Model file for the job. Use its own axes, mm. Face numbers are marked on the shaded views. A direction names the side the tool comes from. Give positions to 0.01 mm unless a question says otherwise; leave off trailing zeros. Loops run counter-clockwise (first coordinate to the right, second up) from the corner with the lowest first, then second, coordinate; pieces in that order, holes last. Notation, with made-up numbers: (23.5, 57.5) - (50.5, 57.5) arc R16 cw to (50.5, 67.5) - close; hole circle Ø2 at (50, -28). An arc over 180 degrees is marked (long way). Use a Markdown table: item, result.
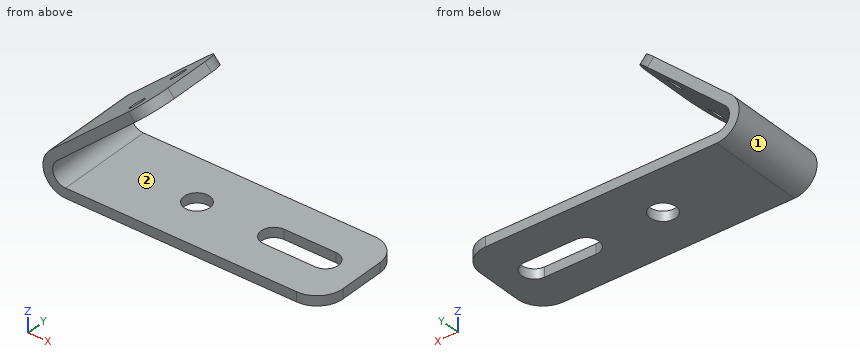
from build123d import *

# Parameters (mm, degrees)
F0_W          = 1270
F0_H          = 48.26
F1_DEPTH      = 483.87
F2_R          = 127
F3_R          = 127
F4_R          = 38.1
F5_DEPTH      = 119.38
F6_R          = 63.5
F7_DEPTH      = 76.2
F7_DEPTH_BACK = 76.2


with BuildPart() as f1:
    # F0 (on Front) → F1 (new body)
    with BuildSketch(Plane.XZ):
        with Locations((271.5897267231, -0.2383861614)):
            Rectangle(F0_W, F0_H)
        with BuildLine():
            Line((-363.4102732769, -24.3683861614), (-363.4102732769, 23.8916138386))
            ThreePointArc((-363.4102732769, 23.8916138386), (-423.8304438336, 67.7016554332), (-400.9706434856, 138.7463335075))
            Line((-400.9706434856, 138.7463335075), (-433.0378788647, 174.8118296935))
            ThreePointArc((-433.0378788647, 174.8118296935), (-468.9099911057, 50.5119834442), (-363.4102732769, -24.3683861614))
        make_face()
        Polygon((-433.0378788647, 174.8118296935), (-400.9706434856, 138.7463335075), (73.5753589619, 560.6836411268), (41.5081235828, 596.7491373128), align=None)
    extrude(amount=F1_DEPTH)

    # F2
    f2_edges = [f1.edges().sort_by_distance(p)[0] for p in [
        (57.541741, 0, 578.716389),
        (57.541741, -483.87, 578.716389),
    ]]
    fillet(f2_edges, radius=F2_R)

    # F3
    f3_edges = [f1.edges().sort_by_distance(p)[0] for p in [
        (906.589727, -483.87, -0.238386),
        (906.589727, 0, -0.238386),
    ]]
    fillet(f3_edges, radius=F3_R)

    # F4 (on face) → F5 (cut)
    with BuildSketch(Plane(origin=(-277.999987923, 0, 312.6620485248), x_dir=(0.7473165393, 0, 0.664468201), z_dir=(-0.664468201, 0, 0.7473165393))):
        with Locations((237.0405329721, -114.3)):
            Circle(F4_R)
        with Locations((237.0405329721, -369.57)):
            Circle(F4_R)
    extrude(amount=-F5_DEPTH, mode=Mode.SUBTRACT)

    # F6 (on face) → F7 (cut, two sides)
    with BuildSketch(Plane.XY.offset(23.8916138386)) as f7_sk:
        with Locations((93.7897267231, -241.935)):
            Circle(F6_R)
        with BuildLine():
            ThreePointArc((538.0487868786, -241.935), (519.4500674839, -197.0337193947), (474.5487868786, -178.435))
            ThreePointArc((474.5487868786, -178.435), (411.0487868786, -241.935), (474.5487868786, -305.435))
            ThreePointArc((474.5487868786, -305.435), (519.4500674839, -286.8362806053), (538.0487868786, -241.935))
        make_face()
        with BuildLine():
            ThreePointArc((729.6141386032, -305.435), (666.1141386032, -241.935), (729.6141386032, -178.435))
            Line((729.6141386032, -178.435), (474.5487868786, -178.435))
            ThreePointArc((474.5487868786, -178.435), (519.4500674839, -197.0337193947), (538.0487868786, -241.935))
            ThreePointArc((538.0487868786, -241.935), (519.4500674839, -286.8362806053), (474.5487868786, -305.435))
            Line((474.5487868786, -305.435), (729.6141386032, -305.435))
        make_face()
        with BuildLine():
            ThreePointArc((729.6141386032, -305.435), (774.5154192086, -286.8362806053), (793.1141386032, -241.935))
            ThreePointArc((793.1141386032, -241.935), (774.5154192086, -197.0337193947), (729.6141386032, -178.435))
            ThreePointArc((729.6141386032, -178.435), (666.1141386032, -241.935), (729.6141386032, -305.435))
        make_face()
    extrude(amount=-F7_DEPTH, mode=Mode.SUBTRACT)
    extrude(f7_sk.sketch, amount=F7_DEPTH_BACK, mode=Mode.SUBTRACT)


solid = f1.part
(1) Drill centre lines: probe 1 along Z at (x, y) = (591.5, -327); probe 2 along Z at (x, y) = (19.5, -57); probe 3 along Z at (x, y) = (-259, -419.5). Where is each one in solid material? Low to high. Write a range as [from, to].
Computed:
| item | result |
|---|---|
| probe 1 | [-24.37, 23.89] |
| probe 2 | [-24.37, 23.89], [512.6, 577.18] |
| probe 3 | [-24.37, 23.89], [264.98, 329.56] |
(2) Pin check, flat tips, straight feed: P1, Ø1, axis at y = -313, z = 426.5, coming from the +X side; P2, Ø1.5, axis at y = -166, z = 165, coming from the -X side; P3, Ø10, axis at x = 562, y = -409, coming from the +Z side. Stop position of each tip, or through.
Computed:
| item | result |
|---|---|
| P1 | x = -76.78 |
| P2 | x = -444.55 |
| P3 | z = 23.89 |
(3) Slice it at A-A, the plane x = 520.5. Write the cut outline in (y, z) (3 decimals).
Computed:
| item | result |
|---|---|
| outline | (-483.87, -24.368) - (-305.435, -24.368) - (-305.435, 23.892) - (-483.87, 23.892) - close; (-178.435, -24.368) - (0, -24.368) - (0, 23.892) - (-178.435, 23.892) - close |
(4) Slice it at C-C, the plane y = -63. Write the cut outline in (x, z).
Computed:
| item | result |
|---|---|
| outline | (-433.04, 174.81) arc R111.76 ccw to (-363.41, -24.37) - (889.28, -24.37) - (889.28, 23.89) - (-363.41, 23.89) arc R63.57 cw to (-400.97, 138.75) - (60.64, 549.19) - (28.58, 585.25) - close |
(5) Slice it at B-B, the plane y = -386. Write the cut outline in (x, z).
Computed:
| item | result |
|---|---|
| outline | (-433.04, 174.81) arc R111.76 ccw to (-363.41, -24.37) - (903.2, -24.37) - (903.2, 23.89) - (-363.41, 23.89) arc R63.57 cw to (-400.97, 138.75) - (-94.48, 411.26) - (-126.54, 447.33) - close; (-75.17, 493.01) - (-43.1, 456.94) - (71.05, 558.43) - (38.98, 594.5) - close |
(6) Slice it at D-D, the plane z = 62.5. Write the cut outline in (x, y), plus the area to 3 significant figures.
Computed:
| item | result |
|---|---|
| outline | (-472.36, -483.87) - (-421.87, -483.87) - (-421.87, 0) - (-472.36, 0) - close |
| area | 24,400 mm² |
(7) 3-axis set-ups, long thin cutter, end or side, ignore diameter. For the marked faces 1 and 2: which of +Z, -Z, +X, -X, +Y, -Y reach the whole face in a straight line?
Computed:
| item | result |
|---|---|
| face 1 | -X, +Y, -Y |
| face 2 | +X, +Y, -Y |
